```python
from build123d import *

# Parameters (mm, degrees)
PAD_DEPTH           = 150
SKETCH001_W         = 32.4797945384
SKETCH001_H         = 60
SKETCH001_W_2       = 36.6107585384
POCKET_DEPTH        = 5
SKETCH007_W         = 10
SKETCH007_H         = 20
PAD001_DEPTH        = 10
SKETCH002_R         = 1.25
HOLE_DEPTH          = 25
HOLE_TIPS_R         = 1.25
HOLE001_D           = 2.5
HOLE001_DEPTH       = 25
HOLE001_CSINK_D     = 6.1
HOLE001_CSINK_ANGLE = 90
HOLE001_TIPS_R      = 1.25
SKETCH006_W         = 74.5044810012
SKETCH006_H         = 25
SKETCH006_W_2       = 72.8484770001
POCKET001_DEPTH     = 11
SKETCH005_W         = 80.411114
SKETCH005_H         = 25
SKETCH005_W_2       = 78.205579
POCKET002_DEPTH     = 11
SKETCH009_W         = 67.6905989232
SKETCH009_H         = 1
PAD002_DEPTH        = 10
HOLE002_D           = 2.5
HOLE002_DEPTH       = 25
HOLE002_CSINK_D     = 6.1
HOLE002_CSINK_ANGLE = 90
HOLE002_TIPS_R      = 1.25


with BuildPart() as part:
    # Sketch → Pad (new body)
    with BuildSketch(Plane.XY):
        Polygon((84.6025403784, 1.1547005384), (0, 50), (-86.6025403784, 0), (-87.6025403784, 1.7320508076), (-69.7820323028, 12.0207259422), (-75.7820323028, 22.4130307876), (-23.8205080757, 52.4130307876), (-17.8205080757, 42.0207259422), (0, 52.3094010768), (17.3205080757, 42.3094010768), (23.3205080757, 52.7017059222), (75.2820323028, 22.7017059222), (69.2820323028, 12.3094010768), (87.6025403784, 1.7320508076), (86.6025403784, 0), (86.6025403784, -15), (84.6025403784, -15), align=None)
        Polygon((-71.6839560914, 21.3149545762), (-69.6839560914, 17.8508529611), (-22.6865334795, 44.4489291724), (-24.6865334795, 47.9130307876), align=None, mode=Mode.SUBTRACT)
        Polygon((69.1839560914, 18.1395280957), (71.1839560914, 21.6036297108), (24.418584287, 48.6036297108), (22.418584287, 45.1395280957), align=None, mode=Mode.SUBTRACT)
    extrude(amount=PAD_DEPTH)

    # Sketch001 (on Face4 of Pad) → Pocket (cut)
    with BuildSketch(Plane(origin=(84.6025403784, 0, 0), x_dir=(0, -1, 0), z_dir=(-1, 0, 0))):
        with Locations((15.0851967308, 30)):
            Rectangle(SKETCH001_W, SKETCH001_H)
        with Locations((17.1506787308, 120)):
            Rectangle(SKETCH001_W_2, SKETCH001_H)
    extrude(amount=-POCKET_DEPTH, mode=Mode.SUBTRACT)

    # Sketch007 (on Face30 of Pocket) → Pad001 (join)
    with BuildSketch(Plane(origin=(84.6025403784, 0, 0), x_dir=(0, -1, 0), z_dir=(-1, 0, 0))):
        with Locations((6.9226497308, 75)):
            Rectangle(SKETCH007_W, SKETCH007_H)
    extrude(amount=PAD001_DEPTH)

    # Sketch002 (on Face5 of Pocket) → Hole (cut)
    with BuildSketch(Plane.YZ.offset(86.6025403784)):
        with Locations((-7.5, 80)):
            Circle(SKETCH002_R)
        with Locations((-7.5, 70)):
            Circle(SKETCH002_R)
    extrude(amount=-HOLE_DEPTH, mode=Mode.SUBTRACT)

    # Hole tips → Hole tip 1 section 0
    with BuildSketch(Plane.YZ.offset(61.6025403784), mode=Mode.PRIVATE) as hole_tip_1_s0:
        with Locations((-7.5, 80)):
            Circle(HOLE_TIPS_R)
    loft([hole_tip_1_s0.sketch, Vertex(60.8514646047, -7.5, 80)], mode=Mode.SUBTRACT)

    # Hole tips → Hole tip 2 section 0
    with BuildSketch(Plane.YZ.offset(61.6025403784), mode=Mode.PRIVATE) as hole_tip_2_s0:
        with Locations((-7.5, 70)):
            Circle(HOLE_TIPS_R)
    loft([hole_tip_2_s0.sketch, Vertex(60.8514646047, -7.5, 70)], mode=Mode.SUBTRACT)

    # Hole001
    with Locations(Plane(origin=(-22.6506350946, 39.2320508076, 0), x_dir=(-0.8660254038, -0.5, 0), z_dir=(-0.5, 0.8660254038, 0))):
        with Locations((67.5, 80), (67.5, 70)):
            CounterSinkHole(HOLE001_D / 2, HOLE001_CSINK_D / 2, depth=HOLE001_DEPTH, counter_sink_angle=HOLE001_CSINK_ANGLE)

    # Hole001 tips → Hole001 tip 1 section 0
    with BuildSketch(Plane(origin=(-10.1506350946, 17.581415713, 0), x_dir=(-0.8660254038, -0.5, 0), z_dir=(-0.5, 0.8660254038, 0)), mode=Mode.PRIVATE) as hole001_tip_1_s0:
        with Locations((67.5, 80)):
            Circle(HOLE001_TIPS_R)
    loft([hole001_tip_1_s0.sketch, Vertex(-68.2318119632, -16.8190349873, 80)], mode=Mode.SUBTRACT)

    # Hole001 tips → Hole001 tip 2 section 0
    with BuildSketch(Plane(origin=(-10.1506350946, 17.581415713, 0), x_dir=(-0.8660254038, -0.5, 0), z_dir=(-0.5, 0.8660254038, 0)), mode=Mode.PRIVATE) as hole001_tip_2_s0:
        with Locations((67.5, 70)):
            Circle(HOLE001_TIPS_R)
    loft([hole001_tip_2_s0.sketch, Vertex(-68.2318119632, -16.8190349873, 70)], mode=Mode.SUBTRACT)

    # Sketch006 (on Face15 of Pocket) → Pocket001 (cut)
    with BuildSketch(Plane(origin=(-28.6506350946, 49.624355653, 0), x_dir=(-0.8660254038, -0.5, 0), z_dir=(-0.5, 0.8660254038, 0))):
        with Locations((24.7169745006, 137.5)):
            Rectangle(SKETCH006_W, SKETCH006_H)
        with Locations((24.0525555, 12.5)):
            Rectangle(SKETCH006_W_2, SKETCH006_H)
    extrude(amount=-POCKET001_DEPTH, mode=Mode.SUBTRACT)

    # Sketch005 (on Face20 of Pocket) → Pocket002 (cut)
    with BuildSketch(Plane(origin=(28.6506350946, 49.624355653, 0), x_dir=(-0.8660254038, 0.5, 0), z_dir=(0.5, 0.8660254038, 0))):
        with Locations((-23.058333, 137.5)):
            Rectangle(SKETCH005_W, SKETCH005_H)
        with Locations((-22.9755485, 12.5)):
            Rectangle(SKETCH005_W_2, SKETCH005_H)
    extrude(amount=-POCKET002_DEPTH, mode=Mode.SUBTRACT)

    # Sketch009 (on Face10 of Pocket) → Pad002 (join)
    with BuildSketch(Plane(origin=(21.6506350946, 37.5, 0), x_dir=(0.8660254038, -0.5, 0), z_dir=(-0.5, -0.8660254038, 0))):
        with Locations((23.8452994616, 21)):
            Rectangle(SKETCH009_W, SKETCH009_H)
    extrude(amount=PAD002_DEPTH)

    # Hole002
    with Locations(Plane(origin=(-23.1506350946, 40.0980762114, 0), x_dir=(-0.8660254038, -0.5, 0), z_dir=(-0.5, 0.8660254038, 0))):
        with Locations((24.9226497308, 145), (24.9226497308, 15)):
            CounterSinkHole(HOLE002_D / 2, HOLE002_CSINK_D / 2, depth=HOLE002_DEPTH, counter_sink_angle=HOLE002_CSINK_ANGLE)

    # Hole002 tips → Hole002 tip 1 section 0
    with BuildSketch(Plane(origin=(-10.6506350946, 18.4474411167, 0), x_dir=(-0.8660254038, -0.5, 0), z_dir=(-0.5, 0.8660254038, 0)), mode=Mode.PRIVATE) as hole002_tip_1_s0:
        with Locations((24.9226497308, 145)):
            Circle(HOLE002_TIPS_R)
    loft([hole002_tip_1_s0.sketch, Vertex(-31.8587450042, 5.3356655511, 145)], mode=Mode.SUBTRACT)

    # Hole002 tips → Hole002 tip 2 section 0
    with BuildSketch(Plane(origin=(-10.6506350946, 18.4474411167, 0), x_dir=(-0.8660254038, -0.5, 0), z_dir=(-0.5, 0.8660254038, 0)), mode=Mode.PRIVATE) as hole002_tip_2_s0:
        with Locations((24.9226497308, 15)):
            Circle(HOLE002_TIPS_R)
    loft([hole002_tip_2_s0.sketch, Vertex(-31.8587450042, 5.3356655511, 15)], mode=Mode.SUBTRACT)


solid = part.part
```
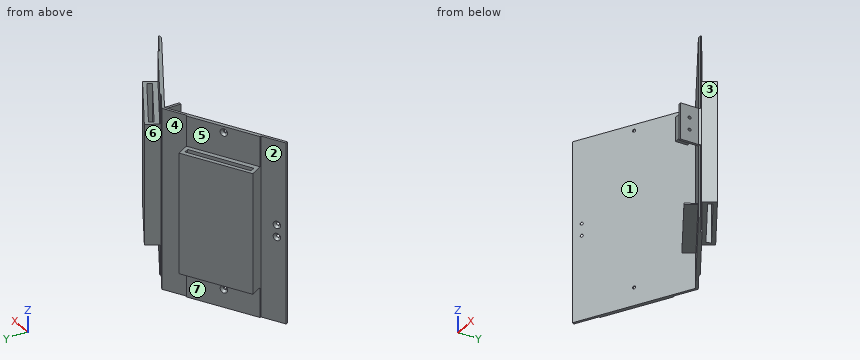
Here's how the part is built. I have some questions about the finished solid (model axes, mm). Face numbers are marked on the shaded views. A direction names the side the tool comes from. Coordinates: 2 decimals unless noted, no trailing zeros. Write each loop counter-clockwise with the first axis right and the second up, starting at its lowest first coordinate (ties: lowest second). Pieces come first, ordered by that corner, then holes. Notation, with made-up numbers: (71.25, 11.25) -> (110.25, 11.25) arc R34 ccw to (110.25, 43.25) -> close; hole circle Ø5 at (12, 81). An arc over 180 degrees is marked (long way). Use a Markdown table: item, result. Add a question column.
(1) We'd pull the mould along Y, two halves only. Please class the marked faces 1, 2, 3 and 4: +Y half, -Y half, draft (parallel to the pull), parting line (faces both ways), or undercut.
(2) For the marked faces 5, 6 and 7, which set-ups out of +Z, -Z, +X, -X, +Y, -Y let a thin tool reach every point of the face, with its end or its side?
(3) Please list where these lines run through material, in increasing order: line 1 (Z direction, x = 82.5, y = -7.5); line 2 (Y direction, x = 80.5, z = 70); line 3 (Z direction, x = 78, y = -7).
(4) I'm going to push flat-ended pins straight in: P1, Ø10, axis at x = -11.5, z = 65, coming from the +Y side; P2, Ø11, axis at x = 77.5, z = 73, coming from the +Y side; P3, Ø2, axis at y = 29.5, z = 78.5, coming from the -X side. Where does each tip first touch, or does it pass through?
(5) If we section it at B-B, the plane x = -36.5: Write out the boundary of the cut face in (y, z).
(6) If we section it at A-A, the plane z = 123: Write out the boundary of the cut face in (x, y), and give its area (3 significant figures).
Outcome:
| question | item | result |
|---|---|---|
| 1 | face 1 | -Y half |
| 1 | face 2 | undercut |
| 1 | face 3 | undercut |
| 1 | face 4 | +Y half |
| 2 | face 5 | +Z, -X, +Y |
| 2 | face 6 | +Z, -Z, +Y |
| 2 | face 7 | -Z, -X, +Y |
| 3 | line 1 | z = 65 to 68.75, 71.25 to 78.75, 81.25 to 85 |
| 3 | line 2 | y = -11.92 to -8.75, -6.25 to -1.92, 3.52 to 5.83 |
| 3 | line 3 | z = 65 to 68.85, 71.15 to 78.85, 81.15 to 85 |
| 4 | P1 | stops at y = 48.56 |
| 4 | P2 | stops at y = 24.6 |
| 4 | P3 | stops at x = -65.24 |
| 5 | outline | (28.93, 0) -> (32.39, 0) -> (32.39, 25) -> (36.63, 25) -> (36.63, 125) -> (32.39, 125) -> (32.39, 150) -> (28.93, 150) -> close; (41.23, 25) -> (45.09, 25) -> (45.09, 125) -> (41.23, 125) -> close |
| 6 | outline | (-87.6, 1.73) -> (-86.6, 0) -> (0, 50) -> (84.6, 1.15) -> (87.27, 1.15) -> (87.6, 1.73) -> (69.28, 12.31) -> (75.28, 22.7) -> (23.32, 52.7) -> (17.32, 42.31) -> (0, 52.31) -> (-17.82, 42.02) -> (-23.82, 52.41) -> (-75.78, 22.41) -> (-69.78, 12.02) -> close; hole (-71.68, 21.31) -> (-69.68, 17.85) -> (-22.69, 44.45) -> (-24.69, 47.91) -> close; hole (22.42, 45.14) -> (69.18, 18.14) -> (71.18, 21.6) -> (24.42, 48.6) -> close |
| 6 | area | 1,410 mm^2 |
